Source: CAD feature listing. Evaluate the final solid. Frame: model axes, mm. A direction names the side the tool comes from. Coordinates: 2 decimals unless noted, no trailing zeros. Order: outer loops, then holes, each group sorted by start corner. A loop starts at its lowest first (then second) coordinate and runs counter-clockwise, first axis right, second up.
Item 1: Mould query, pull axis X, two halves, no side actions, for faces 6 (the cylindrical face through (-21.984, -4.93, -14.382)), 7 (the cylindrical face through (14.77, -4.93, 18.07)), 8 (the cylindrical face through (22.796, -4.93, 6.581)). Classes: released by +X, released by -X, zero draft, split by the parting line, or undercut.
Item 2: Section D-D on y = -6. Return the cut outline in (x, z), then the cut area to 3 significant figures.
Item 3: Section C-C on z = -20.5. Return the cut outline in (x, y).
Item 4: Ray query, line 1 (X direction, y = -7, z = -19); line 2 (X direction, y = -7.5, z = 18); line 3 (X direction, y = -2.5, z = -20). Return the intervals inside material, ascending.
Item 5: Reachability of faces 1 (the flat face through (-19.29, -4.93, -21.126)), 2 (the flat face through (-26.2, -5, 12)), 3 (the flat face through (21.18, -4.93, 14.64)), 4 (the cylindrical face through (-0.661, -9.507, -24.523)), 5 (the flat face through (-23.768, -4.93, -16.275)) from +Z, -Z, +X, -X, +Y, -Y: full face, straight path, thin tool, end or side. Return the list, or none.
Item 6: Section A-A on z = 13. Return the cut outline in (x, y).
Item 7: Contact query for flat-ended pins moving along their axis: P1, Ø1, axis at y = -5, z = 24.5, coming from the -X side; P2, Ø5, axis at x = -15.5, z = 8.5, coming from the -Y side; P3, Ø2.5, axis at x = 20, z = 18, coming from the +Y side; P4, Ø2, axis at x = 11, y = -4.5, coming from the -Z side. Output: stop coordinate, or through.
Item 8: Section B-B on x = -1.2. Return the cut outline in (y, z).
from build123d import *

# Parameters (mm, degrees)
SKETCH_1_R          = 16
SKETCH_1_R_2        = 2.25
EXTRUDE_1_DEPTH     = 10
CUT_EXTRUDE_1_DEPTH = 8.8
CUT_EXTRUDE_8_DEPTH = 1


with BuildPart() as part:
    # Эскиз1 → Бобышка-Вытянуть1 (new body)
    with BuildSketch(Plane(origin=(0, 0, 0), x_dir=(1, 0, 0), z_dir=(0, 1, 0))):
        with BuildLine():
            Line((-26.2, -25), (0.6, -25))
            Line((0.6, -25), (0.6, -24.052407766))
            ThreePointArc((0.6, -24.052407766), (1.160508995, -22.66393175), (2.527865647, -22.05370903))
            ThreePointArc((2.527865647, -22.05370903), (8.609379582, -20.969032322), (14.151976117, -18.241220202))
            ThreePointArc((14.151976117, -18.241220202), (14.777726241, -18.069792078), (15.376980036, -18.318480053))
            Line((15.376980036, -18.318480053), (17.814747272, -20.472785982))
            ThreePointArc((17.814747272, -20.472785982), (22.472785982, -20.185252728), (22.185252728, -15.527214018))
            Line((22.185252728, -15.527214018), (20.143734708, -13.723081814))
            ThreePointArc((20.143734708, -13.723081814), (19.813719174, -13.098302749), (19.979075206, -12.411340949))
            ThreePointArc((19.979075206, -12.411340949), (22.823148445, -6.493089604), (23.8, 0))
            ThreePointArc((23.8, 0), (9.805861096, 22.475890034), (-16.53246264, 19.775101396))
            ThreePointArc((-16.53246264, 19.775101396), (-17.177514672, 19.565457211), (-17.807958535, 19.815623843))
            Line((-17.807958535, 19.815623843), (-20.814747272, 22.472785982))
            ThreePointArc((-20.814747272, 22.472785982), (-25.472785982, 22.185252728), (-25.185252728, 17.527214018))
            Line((-25.185252728, 17.527214018), (-22.311461479, 14.987584542))
            ThreePointArc((-22.311461479, 14.987584542), (-21.982680627, 14.372275298), (-22.136211376, 13.691738288))
            ThreePointArc((-22.136211376, 13.691738288), (-25.166639381, 7.142239829), (-26.2, 0))
            Line((-26.2, 0), (-26.2, -25))
        make_face()
        with Locations(Location((0, 0, 0), (0, 0, 270))):
            Circle(SKETCH_1_R, mode=Mode.SUBTRACT)
        with Locations(Location((-23, 20, 0), (0, 0, 270))):
            Circle(SKETCH_1_R_2, mode=Mode.SUBTRACT)
        with Locations(Location((20, -18, 0), (0, 0, 270))):
            Circle(SKETCH_1_R_2, mode=Mode.SUBTRACT)
    extrude(amount=-EXTRUDE_1_DEPTH)

    # Эскиз2 → Вырез-Вытянуть1 (cut)
    with BuildSketch(Plane(origin=(0, -10, 0), x_dir=(-1, 0, 0), z_dir=(0, -1, 0))):
        with BuildLine():
            Line((0.4, -25), (0.4, -24.052407766))
            ThreePointArc((0.4, -24.052407766), (-0.440763493, -21.969693742), (-2.491798471, -21.054359663))
            ThreePointArc((-2.491798471, -21.054359663), (-8.297732589, -20.018834368), (-13.589169994, -17.414631267))
            ThreePointArc((-13.589169994, -17.414631267), (-16.632858543, -14.893819788), (-19.152217909, -11.84892917))
            ThreePointArc((-19.152217909, -11.84892917), (-21.867498452, -6.198584635), (-22.799999992, 0.0005752))
            ThreePointArc((-22.799999992, 0.0005752), (-9.365885893, 21.577880063), (15.919164541, 18.985249865))
            ThreePointArc((15.919164541, 18.985249865), (18.852153178, 16.289251545), (21.298763477, 13.145221119))
            ThreePointArc((21.298763477, 13.145221119), (24.208055551, 6.857429147), (25.2, 0.000581878))
            Line((25.2, 0.000581878), (25.2, -25))
            Line((25.2, -25), (0.4, -25))
        make_face()
    extrude(amount=-CUT_EXTRUDE_1_DEPTH, mode=Mode.SUBTRACT)

    # Эскиз11 → Вырез-Вытянуть8 (cut)
    with BuildSketch(Plane.XZ.offset(10)):
        with BuildLine():
            Line((-0.4, 24.052407766), (-0.4, 25))
            Line((-0.4, 25), (0.1, 25))
            Line((0.1, 25), (0.1, 24.052407766))
            ThreePointArc((0.1, 24.052407766), (0.800636244, 22.316812746), (2.509832059, 21.554034346))
            ThreePointArc((2.509832059, 21.554034346), (17.255552057, 14.973268455), (23.299999998, -0.000287804))
            ThreePointArc((23.299999998, -0.000287804), (-1.199999175, -24.528816589), (-25.7, -0.000289454))
            Line((-25.7, -0.000289454), (-25.7, 25))
            Line((-25.7, 25), (-25.2, 25))
            Line((-25.2, 25), (-25.2, -0.000581878))
            ThreePointArc((-25.2, -0.000581878), (-1.199996661, -24.028816589), (22.799999992, -0.0005752))
            ThreePointArc((22.799999992, -0.0005752), (16.895779065, 14.626046024), (2.491798471, 21.054359663))
            ThreePointArc((2.491798471, 21.054359663), (0.440763493, 21.969693742), (-0.4, 24.052407766))
        make_face()
    extrude(amount=-CUT_EXTRUDE_8_DEPTH, mode=Mode.SUBTRACT)


solid = part.part
Answer list:
1. face 6: released by -X
1. face 7: undercut
1. face 8: released by +X
2. outline: (-26.2, 0) arc R25 ccw to (-22.14, -13.69) arc R1 cw to (-22.31, -14.99) - (-25.19, -17.53) arc R3.3 ccw to (-20.81, -22.47) - (-17.81, -19.82) arc R1 cw to (-16.53, -19.78) arc R25 ccw to (23.8, 0) arc R22.07 ccw to (19.98, 12.41) arc R1 cw to (20.14, 13.72) - (22.19, 15.53) arc R3.3 ccw to (17.81, 20.47) - (15.38, 18.32) arc R1 cw to (14.15, 18.24) arc R22.07 ccw to (2.53, 22.05) arc R2 cw to (0.6, 24.05) - (0.6, 25) - (-0.4, 25) - (-0.4, 24.05) arc R3 ccw to (2.49, 21.05) arc R21.07 cw to (22.8, 0) arc R24 cw to (-25.2, 0) - (-25.2, 25) - (-26.2, 25) - close; hole circle Ø4.5 at (-23, -20); hole circle Ø4.5 at (20, 18)
2. area: 198 mm2
3. outline: (-26.26, -10) - (-25.19, -10) - (-25.19, 0) - (-26.26, 0) - close; (-20.81, -10) - (-18.58, -10) - (-18.58, 0) - (-20.81, 0) - close; (-15.55, -10) - (-14.66, -10) - (-14.66, -9) - (-13.73, -9) - (-13.73, -1.2) - (11.33, -1.2) - (11.33, -9) - (12.26, -9) - (12.26, -10) - (13.15, -10) - (13.15, 0) - (-15.55, 0) - close
4. line 1: x = -26.14 to -25.02, -20.98 to -15.9, 13.5 to 15.08
4. line 2: x = -26.2 to -25.2, 12.68 to 17.75, 22.25 to 23.3
4. line 3: x = -26.3 to -25.25, -20.75 to -18.02, -16.24 to -14.51, 12.11 to 13.84
5. face 1: -Z, +Y, -Y
5. face 2: +Z, -X, +Y, -Y
5. face 3: +X, +Y, -Y
5. face 4: -Y
5. face 5: -X, +Y, -Y
6. outline: (-26.2, -10) - (-25.7, -10) - (-25.7, -9) - (-25.2, -9) - (-25.2, -1.2) - (-9.33, -1.2) - (-9.33, 0) - (-26.2, 0) - close; (9.33, -1.2) - (18.31, -1.2) - (18.31, -9) - (18.94, -9) - (18.94, -10) - (19.81, -10) - (19.81, 0) - (9.33, 0) - close
7. P1: stops at x = -26.2
7. P2: stops at y = -1.2
7. P3: passes through
7. P4: stops at z = -22.38
8. outline: (-10, -25.03) - (0, -25.03) - (0, -15.95) - (-1.2, -15.95) - (-1.2, -24.03) - (-9, -24.03) - (-9, -24.53) - (-10, -24.53) - close; (-1.2, 15.95) - (0, 15.95) - (0, 25) - (-1.2, 25) - close
